```python
from build123d import *

# Parameters (mm, degrees)
EXTRUDE_1_DEPTH      = 16
SKETCH_2_R           = 16
CUT_EXTRUDE_1_DEPTH  = 15
SKETCH_3_R           = 13
CUT_EXTRUDE_2_DEPTH  = 120.713198938
SKETCH_4_R           = 20.5
CUT_EXTRUDE_3_DEPTH  = 5
HOLE_WIZARD_M32_D    = 3.4
CUT_EXTRUDE_8_DEPTH  = 30
CUT_EXTRUDE_11_DEPTH = 120.842605112
EXTRUDE_2_DEPTH      = 11
FILLET_1_R           = 4
M4X0_71_D            = 3.3


with BuildPart() as part:
    # Эскиз1 → Бобышка-Вытянуть1 (new body)
    with BuildSketch(Plane(origin=(0, 0, 0), x_dir=(1, 0, 0), z_dir=(0, 1, 0))):
        with BuildLine():
            Line((0, 0), (0, 60))
            Line((0, 60), (-30, 60))
            Line((-30, 60), (-83.234756238, 52.266260397))
            ThreePointArc((-83.234756238, 52.266260397), (-102.5, 30), (-83.234756238, 7.733739603))
            Line((-83.234756238, 7.733739603), (-30, 0))
            Line((-30, 0), (0, 0))
        make_face()
    extrude(amount=EXTRUDE_1_DEPTH)

    # Эскиз2 → Вырез-Вытянуть1 (cut)
    with BuildSketch(Plane.XZ):
        with Locations(Location((-80, -30, 0), (0, 0, 270))):
            Circle(SKETCH_2_R)
    extrude(amount=-CUT_EXTRUDE_1_DEPTH, mode=Mode.SUBTRACT)

    # Эскиз3 → Вырез-Вытянуть2 (cut, through all)
    with BuildSketch(Plane.XZ.offset(-15)):
        with Locations(Location((-80, -30, 0), (0, 0, 270))):
            Circle(SKETCH_3_R)
    extrude(amount=-CUT_EXTRUDE_2_DEPTH, mode=Mode.SUBTRACT)

    # Эскиз4 → Вырез-Вытянуть3 (cut)
    with BuildSketch(Plane.XZ):
        with Locations(Location((-80, -30, 0), (0, 0, 270))):
            Circle(SKETCH_4_R)
    extrude(amount=-CUT_EXTRUDE_3_DEPTH, mode=Mode.SUBTRACT)

    # Отверстие с зазором M32 (through all)
    with Locations(Plane(origin=(0, 5, 0), x_dir=(-1, 0, 0), z_dir=(0, -1, 0))):
        with Locations((92.904698757, 17.095301243), (67.095301243, 17.095301243), (67.095301243, 42.904698757), (92.904698757, 42.904698757), (80, 11.75), (61.75, 30), (80, 48.25), (98.25, 30)):
            Hole(HOLE_WIZARD_M32_D / 2)

    # Эскиз8 → Вырез-Вытянуть8 (cut)
    with BuildSketch(Plane(origin=(0, 0, 0), x_dir=(0, 0, -1), z_dir=(1, 0, 0))):
        with BuildLine():
            Line((37.9, 5.9), (22.1, 5.9))
            ThreePointArc((22.1, 5.9), (15.1, 12.9), (8.1, 5.9))
            Line((8.1, 5.9), (0, 5.9))
            Line((0, 5.9), (0, 0))
            Line((0, 0), (60, 0))
            Line((60, 0), (60, 5.9))
            Line((60, 5.9), (51.9, 5.9))
            ThreePointArc((51.9, 5.9), (44.9, 12.9), (37.9, 5.9))
        make_face()
    extrude(amount=-CUT_EXTRUDE_8_DEPTH, mode=Mode.SUBTRACT)

    # Эскиз14 → Вырез-Вытянуть11 (cut, through all)
    with BuildSketch(Plane.XZ):
        with BuildLine():
            Line((-33, -56.53267916), (-76.544602266, -50.206687668))
            ThreePointArc((-76.544602266, -50.206687668), (-59.5, -30), (-76.544602266, -9.793312332))
            Line((-76.544602266, -9.793312332), (-33, -3.46732084))
            Line((-33, -3.46732084), (-33, -56.53267916))
        make_face()
    extrude(amount=-CUT_EXTRUDE_11_DEPTH, mode=Mode.SUBTRACT)

    # Эскиз15 → Бобышка-Вытянуть2 (add, through all)
    with BuildSketch(Plane.XZ.offset(-5)):
        with BuildLine():
            Line((-59.5549517, -31.5), (-33, -31.5))
            Line((-33, -31.5), (-33, -28.5))
            Line((-33, -28.5), (-59.5549517, -28.5))
            ThreePointArc((-59.5549517, -28.5), (-59.5, -30), (-59.5549517, -31.5))
        make_face()
    extrude(amount=-EXTRUDE_2_DEPTH)

    # Скругление1
    fillet_1_edges = [part.edges().sort_by_distance(p)[0] for p in [
        (-76.544602266, 10.5, -50.206687668),
        (-76.544602266, 10.5, -9.793312332),
        (-33, 8, -3.46732084),
        (-33, 8, -56.53267916),
        (-33, 10.5, -28.5),
        (-33, 10.5, -31.5),
        (-59.5549517, 10.5, -31.5),
        (-59.5549517, 10.5, -28.5),
    ]]
    fillet(fillet_1_edges, radius=FILLET_1_R)

    # Отверстие обработанное метчиком M4x0.71 (through all)
    with Locations(Plane(origin=(-72.539630463, 5.9, -28.004308474), x_dir=(-0.7071067811865468, 0, 0.7071067811865482), z_dir=(0, -1, 0))):
        with Locations((-67.376897326, -28.138564072), (-53.234761703, -13.996428448), (-35.026762087, -32.204428064), (-49.168897711, -46.346563688), (-30.960898095, -64.554563303), (-16.818762471, -50.412427679)):
            Hole(M4X0_71_D / 2)


solid = part.part
```
Geometry check sheet. Reference: the model listing, model coordinates, mm. A direction names the side the tool comes from. Coordinates: 2 decimals unless noted, no trailing zeros. Write each loop counter-clockwise with the first axis right and the second up, starting at its lowest first coordinate (ties: lowest second). Pieces come first, ordered by that corner, then holes. Notation, with made-up numbers: (53.5, -30) -> (108.5, -30) arc R13 cw to (108.5, -24) -> close; hole circle Ø4 at (27, 38). An arc over 180 degrees is marked (long way). Use CSV: the item, a comma, the result in double quotes. Start each with the question number.
Item 1: Thickness scan on line 1 (X direction, y = 13.5, z = -30); line 2 (Z direction, x = -5, y = 13); line 3 (X direction, y = 11.5, z = -16.5). Record the ranges inside material, lowest first.
Item 2: Depth check by flat-ended pin: pin 1 Ø1 at (x, y) = (-75, 10.5) entering from -Z; pin 2 Ø1.5 at (x, z) = (-70.5, -44.5) entering from -Y; pin 3 Ø1 at (y, z) = (1.5, -38) entering from +X. Enter the tip coordinate at first touch or a pass-through.
Item 3: Cross-section at B-B, the plane x = -5. Record the cut outline in (y, z).
Item 4: Cross-section at D-D, the plane x = -98.25. Record the cut outline in (y, z), plus the area to 3 significant figures.
Item 5: Cross-section at C-C, the plane y = 2.5. Record the cut outline in (x, z), plus the area to 3 significant figures.
Item 6: Mould release check, pull along Z, two halves, no side actions. Record for faces 5 (the flat face through (-66, 0, -8)), 6 (the flat face through (-56.99, 7.89, -3.92)), 7 (the cylindrical face through (-25.36, 11.02, -57.36)), 8 (the flat face through (-56.245, 7.888, -56.187)): released by +Z, released by -Z, zero draft, split by the parting line, or undercut.
Item 7: Cross-section at A-A, the plane z = -11.75. Record the cut outline in (x, y).
Item 8: Set-up check for faces 1 (the cylindrical face through (-14.79, 12.9, -45.05)), 2 (the flat face through (-15, 5.9, -4)), 3 (the flat face through (-66.9, 15, -28.7)), 4 (the cylindrical face through (-62.247, 10.423, -19.75)): record each of +Z, -Z, +X, -X, +Y, -Y from which the full face is reachable in a straight line by a thin tool's end or side.
Answers:
1,line 1,"-102.5 to -99.95, -96.55 to -96, -64 to -63.45, -60.05 to -26.65, -23.35 to -6.65, -3.35 to 0"
1,line 2,"-60 to -57.4, -54.1 to -31.65, -28.35 to -5.9, -2.6 to 0"
1,line 3,"-98 to -94.5, -91.31 to -88.59, -71.41 to -68.69, -65.5 to -64.57, -33 to -30"
2,pin 1,"z = -53.54"
2,pin 2,"y = 5"
2,pin 3,"x = -30"
3,outline,"(5.9, -60) -> (16, -60) -> (16, -57.4) -> (5.9, -57.4) -> close; (5.9, -54.1) -> (16, -54.1) -> (16, -31.65) -> (5.9, -31.65) -> (5.9, -37.9) arc R7 cw to (5.9, -51.9) -> close; (5.9, -28.35) -> (16, -28.35) -> (16, -5.9) -> (5.9, -5.9) -> (5.9, -8.1) arc R7 cw to (5.9, -22.1) -> close; (5.9, -2.6) -> (16, -2.6) -> (16, 0) -> (5.9, 0) -> close"
4,outline,"(0, -43.16) -> (16, -43.16) -> (16, -31.7) -> (5, -31.7) -> (5, -39.34) -> (0, -39.34) -> close; (0, -20.66) -> (5, -20.66) -> (5, -28.3) -> (16, -28.3) -> (16, -16.84) -> (0, -16.84) -> close"
4,area,"290 mm^2"
5,outline,"(-83.23, -52.27) -> (-30, -60) -> (-30, 0) -> (-83.23, -7.73) arc R22.5 ccw to start; hole (-76.54, -50.21) -> (-37.58, -55.87) arc R4 ccw to (-33, -51.91) -> (-33, -8.09) arc R4 ccw to (-37.58, -4.13) -> (-76.54, -9.79) arc R20.5 ccw (long way) to start"
5,area,"606 mm^2"
6,face 5,"zero draft"
6,face 6,"released by +Z"
6,face 7,"undercut"
6,face 8,"released by -Z"
7,outline,"(-93.16, 0) -> (-89.34, 0) -> (-89.34, 5) -> (-81.7, 5) -> (-81.7, 16) -> (-93.16, 16) -> close; (-78.3, 5) -> (-67.45, 5) -> (-67.45, 16) -> (-78.3, 16) -> close; (-33, 0) -> (-30, 0) -> (-30, 12.05) -> (0, 12.05) -> (0, 16) -> (-33, 16) -> close"
8,face 1,"+X, -Y"
8,face 2,"+Z, -Z, +X, -Y"
8,face 3,"-Y"
8,face 4,"+Y, -Y"
